Source: CAD feature listing. Evaluate the final solid. Frame: model axes, mm. A direction names the side the tool comes from. Give positions to 0.01 mm unless a question says otherwise; leave off trailing zeros. Order: outer loops, then holes, each group sorted by start corner. A loop starts at its lowest first (then second) coordinate and runs counter-clockwise, first axis right, second up. Notation, with made-up numbers: M 33,18.5 L 91,18.5 A16 ccw 91,43.5 Z; hole C 76,-3.75 d2. An arc over 180 degrees is marked long. Return JSON: item names as keys, results as strings.
Autodesk Inventor part; units mm, degrees
ref_plane "IDS_WORKPLANE{1}" through (-5.4864, 0, 0) normal (1, 0, 0) x (0, 0, -1)
ref_plane "Work Plane2" through (41.275, 0, 0) normal (0, 0, -1) x (1, 0, 0)
ref_plane "YZ Plane" through (0, 0, 0) normal (1, 0, 0) x (0, 1, 0)
sketch "Sketch1" plane through (0, 0, 0) normal (0, 0, 1) x (1, 0, 0)
  line L0 (-5.4864, 0) -> (15.875, 0)
  line L1 (15.875, 0) -> (15.875, 3.175)
  line L2 (15.875, 3.175) -> (3.175, 3.175)
  line L3 (3.175, 3.175) -> (2.413, 3.175)
  line L4 (2.413, 3.175) -> (0, 3.175)
  line L5 (0, 3.175) -> (0, 4.7625)
  line L6 (-10.1349, 0) -> (20.21, 0)
  line L7 (0, -0.9693) -> (0, 5.8158)
  line L8 (0, 4.7625) -> (-4.2103, 4.7625)
  arc A0 (-4.2103, 4.7625) -> (-5.4864, 0) centre (4.0386, 0) ccw
  line L9 (3.175, 3.175) -> (0, 3.175) construction
  dimension "d0" = 15.875
  dimension "d1" = 12.7
  dimension "d2" = 0.762
  dimension "d3" = 5.4864
  dimension "d4" = 6.35
  dimension "d5" = 6.35
  dimension "d9" = 9.525
  dimension "d10" = 0
  dimension "d13" = 9.525
revolve "Body" add sketch "Sketch1" angle 360 about axis through (-5.4864, 0, 0) along (1, 0, 0)
ref_plane "IDS_WORKPLANE{1}" through (-5.4864, 0, 0) normal (1, 0, 0) x (0, 0, -1)
sketch "Sketch2" plane through (-5.4864, 0, 0) normal (1, 0, 0) x (0, 0, -1)
  circle A0 centre (0, 0) radius 4.7625
  line L0 (0, -6.6675) -> (0, 6.6675)
  line L1 (6.6675, 0) -> (-6.6675, 0)
  line L2 (-4.7625, 0.9525) -> (4.7625, 0.9525)
  line L3 (4.7625, 0.9525) -> (4.7625, -0.9525)
  line L4 (4.7625, -0.9525) -> (-4.7625, -0.9525)
  line L5 (-4.7625, -0.9525) -> (-4.7625, 0.9525)
  line L6 (-4.7625, 0) -> (4.7625, 0) construction
  line L7 (0, 0.9525) -> (0, -0.9525) construction
  dimension "d15" = 1.905
extrude "Slot" cut sketch "Sketch2" along normal blind 2.4638 contours L1 L0 L2 A0 | L3 L4 A0 | A0 L4 L0 L1 | A0 L2 L3 | L1 A0 L2 L0 | L0 L4 A0 L1 | L5 L2 A0 | A0 L4 L5
thread "Thread"
sketch "Sketch3" plane through (0, 0, 0) normal (0, 0, 1) x (1, 0, 0)
  line L0 (15.875, 0) -> (15.875, 3.175)
  line L1 (15.875, 3.175) -> (3.175, 3.175)
  line L2 (-5.4864, 0) -> (15.875, 0)
  arc A0 (15.875, 0) -> (15.0243, 3.175) centre (9.525, 0) ccw
  line L3 (15.875, -3.175) -> (15.875, 3.175)
  line L4 (15.0243, 3.175) -> (15.0243, 0)
  line L5 (15.0243, 0) -> (15.875, 0)
  dimension "d40" = 6.35
revolve "Fillet1" cut sketch "Sketch3" angle 360 about axis through (-5.4864, 0, 0) along (1, 0, 0) contours A0 L1 L0
chamfer "Chamfer" distance 0.635 angle 45 1 edges at (15.0243, -3.175, 0)
ref_plane "Work Plane2" through (41.275, 0, 0) normal (0, 0, -1) x (1, 0, 0)
fillet "Fillet4" radius 0.7874 1 edges at (0, -3.175, 0)
equation "\"d0\" = NLG"
equation "\"d1\" = GEL"
equation "\"d2\" = GAL"
equation "\"d3\" = KOH"
equation "\"d4\" = GD"
equation "\"d5\" = BDM"
equation "\"d9\" = KOD"
equation "\"d13\" = KR"
equation "\"d15\" = SBR"
equation "\"d16\" = STI"
equation "\"d40\" = GD"
equation "\"d46\" = R"
equation "\"d11\" = GEL"
equation "\"d43\" = 0.5 * RR"
equation "\"GD\" = NND"
equation "\"NLG\" = 15.875"
equation "\"GEL\" = 12.7"
equation "\"KOD\" = 9.525"
equation "\"KOH\" = 5.4864"
equation "\"GAL\" = 0.762"
equation "\"BDM\" = NND"
equation "\"SBR\" = 1.905"
equation "\"STI\" = 2.4638"
equation "\"KEWI\" = 0"
equation "\"KR\" = KOD"
equation "\"d14\" = -KOH"
equation "\"R\" = 0.7874"
equation "\"THREADDIA\" = 6.35"
equation "\"TOA\" = 30deg"
equation "\"KOH1\" = 4.3688"
equation "\"NND\" = 6.35"
equation "\"GD1\" = 4.8387"
equation "\"THREADDESC\" = 1.2345"
properties part number "ANSI B18.6.2 - 1/4-20 UNC - 0.625, SFHCSI" material "Steel, Mild"
1. Section query A-A (x = -3.75). Return loops of the section in (y, z) (1 decimal).
Evaluation:
{"outline": "M -1,-4.7 L -1,4.7 A4.8 ccw Z; M 1,-4.7 A4.8 ccw 1,4.7 Z"}
2. Draft query along Y for faces 3 (the face through (-2.13, -1.03, 4.65)), 4 (the face through (-4, -0.952, 0)), 5 (the face through (0, -2, 4)). Return one class per face: pulls with the +Y half, pulls with the -Y half, needs draft (parallel to the pull), parting line crosses it, or undercut.
Evaluation:
{"face 3": "parting line crosses it", "face 4": "undercut", "face 5": "needs draft"}
3. Set-up query: faces 1 (the face through (-3.023, 0, 0)), 2 (the face through (7.49, -0.69, 3.1)). Return all of +Z, -Z, +X, -X, +Y, -Y with unobstructed straight access to the full face (end or side cutting, diameter ignored); none if empty.
Evaluation:
{"face 1": "+Z, -Z, -X", "face 2": "+X"}
4. Ray query, probe 1 along X at (y, z) = (-4, 1.5); probe 2 along X at (y, z) = (1.25, -2); probe 3 along Z at (x, y) = (3.25, -0.25). Return the intervals inside material, ascending.
Evaluation:
{"probe 1": "x = -4.47 to 0", "probe 2": "x = -5.19 to 15.42", "probe 3": "z = -3.17 to 3.17"}
5. First-contact query: pin 1 (1.5 mm diameter, centred on y = 0, z = 0, fed in from -X); pin 2 (4 mm diameter, centred on y = 3.5, z = -1.5, fed in from +X); pin 3 (1.5 mm diameter, centred on x = -2, z = 2, fed in from -Y). Flat tips, straight axial feed; report the tip coordinate or a pass-through.
Evaluation:
{"pin 1": "stops at x = -3.02", "pin 2": "stops at x = 15.61", "pin 3": "stops at y = -4.6"}
